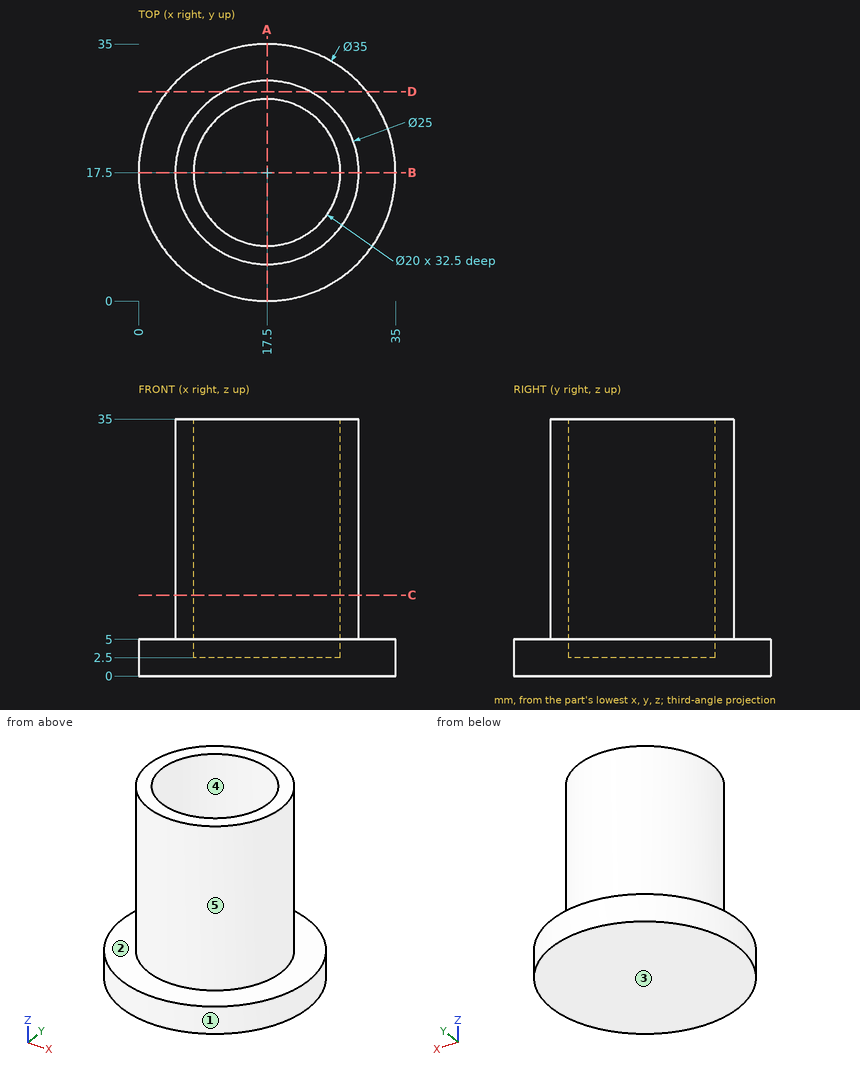
Could you check a few things on this drawing? It's one solid part, dimensions in mm from its lowest x, y, z. A direction names the side the tool comes from. Coordinates: 2 decimals unless noted, no trailing zeros. Loops run counter-clockwise (first coordinate to the right, second up) from the corner with the lowest first, then second, coordinate; pieces in that order, holes last.
1. Imagine slicing it at C-C (z = 11). Please give me the cut outline in (x, y).
2. I need wall thicknesses on L1, parallel to Y at x = 17.5, z = 24; L2, parallel to X at y = 15.5, z = 29.5; L3, parallel to X at y = 10.5, z = 25.5. Which ranges of each line are inside material? Lowest first, please.
3. For P1, Ø2, axis at y = 19.5, z = 24, coming from the -X side; P2, Ø4, axis at x = 28.5, z = 15.5, coming from the -Y side; P3, Ø1.5, axis at y = 10.5, z = 23, coming from the +X side, each with a flat end and sliding along its axis, tell me the tip position at first contact or that it passes through.
4. Imagine slicing it at D-D (y = 28.5). Please give me the cut outline in (x, z), and give its area (3 significant figures).
5. Imagine slicing it at A-A (x = 17.5). Please give me the cut outline in (y, z).
6. For the marked faces 1 and 2, which set-ups out of +Z, -Z, +X, -X, +Y, -Y let a thin tool reach every point of the face, with its end or its side?
7. We'd pull the mould along X, two halves only. Please class the marked faces 3, 4 and 5: released by +X, released by -X, zero draft, split by the parting line, or undercut.
Computed values:
1. outline: circle Ø25 at (17.5, 17.5); hole circle Ø20 at (17.5, 17.5)
2. L1: y = 5 to 7.5, 27.5 to 30
2. L2: x = 5.16 to 7.7, 27.3 to 29.84
2. L3: x = 7.14 to 10.36, 24.64 to 27.86
3. P1: stops at x = 5.04
3. P2: stops at y = 8.83
3. P3: stops at x = 28.33
4. outline: (3.89, 0) - (31.11, 0) - (31.11, 5) - (23.44, 5) - (23.44, 35) - (11.56, 35) - (11.56, 5) - (3.89, 5) - close
4. area: 492 mm2
5. outline: (0, 0) - (35, 0) - (35, 5) - (30, 5) - (30, 35) - (27.5, 35) - (27.5, 2.5) - (7.5, 2.5) - (7.5, 35) - (5, 35) - (5, 5) - (0, 5) - close
6. face 1: +Z, -Z
6. face 2: +Z
7. face 3: zero draft
7. face 4: undercut
7. face 5: split by the parting line
